```python
from build123d import *

# Parameters (mm, degrees)
SKETCH1_W                 = 38.1
SKETCH1_H                 = 41.925
SKETCH1_R                 = 7.5875
BOSS_EXTRUDE1_DEPTH       = 4.826
F_3_0_3_DIAMETER_HOLE1_D  = 3
CHAMFER1_SIZE             = 9.525
CHAMFER2_SIZE             = 3.175
F_4_40_TAPPED_HOLE1_D     = 2.2606
F_4_40_TAPPED_HOLE1_DEPTH = 7.62
F_4_40_TAPPED_HOLE1_TIP   = 0.679152758
F_4_40_TAPPED_HOLE2_D     = 2.2606
F_4_40_TAPPED_HOLE2_DEPTH = 7.62
F_4_40_TAPPED_HOLE2_TIP   = 0.679152758


with BuildPart() as part:
    # Sketch1 → Boss-Extrude1 (new body)
    with BuildSketch(Plane(origin=(0, 0, 0), x_dir=(0, 0, -1), z_dir=(1, 0, 0))):
        with Locations((4.25291004, 9.319846416)):
            Rectangle(SKETCH1_W, SKETCH1_H)
        with Locations(Location((4.25291004, 4.232346416, 0), (0, 0, 90))):
            Circle(SKETCH1_R, mode=Mode.SUBTRACT)
    extrude(amount=BOSS_EXTRUDE1_DEPTH)

    # Ø3.0 (3) Diameter Hole1 (through all)
    with Locations(Plane.ZY):
        with Locations((3.49708996, 24.655740175), (9.576406646, 4.232346416), (-18.082226726, 4.232346416)):
            Hole(F_3_0_3_DIAMETER_HOLE1_D / 2)

    # Chamfer1
    chamfer1_edges = [part.edges().sort_by_distance(p)[0] for p in [
        (2.413, 30.282346416, 14.79708996),
        (2.413, 30.282346416, -23.30291004),
    ]]
    chamfer(chamfer1_edges, length=CHAMFER1_SIZE)

    # Chamfer2
    chamfer2_edges = [part.edges().sort_by_distance(p)[0] for p in [
        (2.413, -11.642653584, -23.30291004),
        (2.413, -11.642653584, 14.79708996),
    ]]
    chamfer(chamfer2_edges, length=CHAMFER2_SIZE)

    # #4-40 Tapped Hole1
    with Locations(Plane(origin=(-40.959349893, -24.044697485, -23.30291004), x_dir=(-1, 0, 0), z_dir=(0, 0, -1))):
        with Locations((-43.372349893, 31.452043901), (-43.372349893, 21.927043901)):
            Hole(F_4_40_TAPPED_HOLE1_D / 2, depth=F_4_40_TAPPED_HOLE1_DEPTH)
            with Locations((0, 0, -(F_4_40_TAPPED_HOLE1_DEPTH + F_4_40_TAPPED_HOLE1_TIP / 2))):  # 118° drill point
                Cone(0, F_4_40_TAPPED_HOLE1_D / 2, F_4_40_TAPPED_HOLE1_TIP, mode=Mode.SUBTRACT)

    # #4-40 Tapped Hole2
    with Locations(Plane(origin=(-40.959349893, -24.044697485, 14.79708996), x_dir=(1, 0, 0), z_dir=(0, 0, 1))):
        with Locations((43.372349893, 21.927043901), (43.372349893, 31.452043901)):
            Hole(F_4_40_TAPPED_HOLE2_D / 2, depth=F_4_40_TAPPED_HOLE2_DEPTH)
            with Locations((0, 0, -(F_4_40_TAPPED_HOLE2_DEPTH + F_4_40_TAPPED_HOLE2_TIP / 2))):  # 118° drill point
                Cone(0, F_4_40_TAPPED_HOLE2_D / 2, F_4_40_TAPPED_HOLE2_TIP, mode=Mode.SUBTRACT)


solid = part.part
```
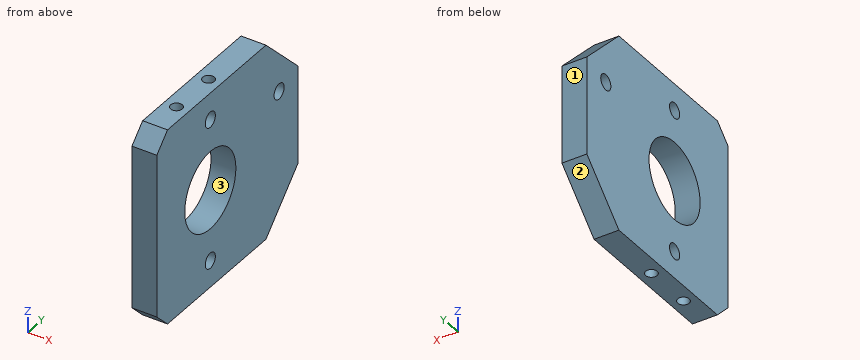
Could you check a few things on this model? Use its own coordinates, in mm. Face numbers are marked on the shaded views. Give positions to 0.01 mm unless a question says otherwise; leave off trailing zeros. Order: outer loops, then holes, each group sorted by start corner. A loop starts at its lowest first (then second) coordinate and runs counter-clockwise, first axis right, second up.
Q1. Suppose I cut it at C-C, the plane x = 4.1. Write out the boundary of the cut face in (y, z) (1 decimal), and give its area (3 significant figures).
Q2. Suppose I cut it at B-B, the plane y = 10. Write out the boundary of the cut face in (x, z).
Q3. If I drill on line 1 along Y through (x, z) = (3.05, 2.5); line 2 along Z through (x, y) = (3.4, 5); line 3 along Y through (x, z) = (2.7, 8), over which ranges is the centre line in solid material (lowest first)?
Q4. I'm going to push a flat-ended pin straight in: P1, Ø2, axis at x = 2.41, y = -2.12, coming from the -Z side. Where does the tip first touch, or does it pass through?
Q5. Suppose I cut it at A-A, the plane z = -7. Write out the boundary of the cut face in (x, y).
Q6. We'd pull the mould along Z, two halves only. Please class the marked faces 1, 2 and 3: +Z half, -Z half, draft (parallel to the pull), parting line (faces both ways), or undercut.
Q7. Suppose I cut it at D-D, the plane z = 6. Write out the boundary of the cut face in (x, y), and give its area (3 significant figures).
Solution:
1. outline: (-11.6, -20.1) - (-8.5, -23.3) - (20.8, -23.3) - (30.3, -13.8) - (30.3, 5.3) - (20.8, 14.8) - (-8.5, 14.8) - (-11.6, 11.6) - close; hole circle Ø15.2 at (4.2, -4.3); hole circle Ø3 at (4.2, -18.1); hole circle Ø3 at (4.2, 9.6); hole circle Ø3 at (24.7, 3.5)
1. area: 1,290 mm2
2. outline: (0, -23.3) - (4.83, -23.3) - (4.83, -9.18) - (0, -9.18) - close; (0, 0.68) - (4.83, 0.68) - (4.83, 14.8) - (0, 14.8) - close
3. line 1: y = -11.64 to 0.77, 7.69 to 23.54, 25.78 to 30.28
3. line 2: z = -23.3 to -19.37, -16.79 to -11.8, 3.3 to 8.29, 10.87 to 14.8
3. line 3: y = -11.64 to -3.21, -1.02 to 6.31, 8.5 to 27.55
4. P1: stops at z = -15.61
5. outline: (0, -11.64) - (4.83, -11.64) - (4.83, -2.84) - (0, -2.84) - close; (0, 11.31) - (4.83, 11.31) - (4.83, 30.28) - (0, 30.28) - close
6. face 1: draft
6. face 2: -Z half
6. face 3: undercut
7. outline: (0, -11.64) - (4.83, -11.64) - (4.83, 29.55) - (0, 29.55) - close
7. area: 199 mm2
